Model file for the job. Use its own axes, mm. A direction names the side the tool comes from. Give positions to 0.01 mm unless a question says otherwise; leave off trailing zeros. Loops run counter-clockwise (first coordinate to the right, second up) from the corner with the lowest first, then second, coordinate; pieces in that order, holes last. Notation, with made-up numbers: M 86,33 L 104,33 A10 cw 104,37 Z; hole C -15.75,12 d10. An arc over 180 degrees is marked long. Use CSV: the item, a comma, the result in double quotes. Start each with the question number.
(1) Flat gauge pins, fed straight in: P1, Ø3, axis at y = 4, z = -2, coming from the -X side; P2, Ø3, axis at y = 4, z = -4, coming from the +X side; P3, Ø1.5, axis at x = 14.5, z = -34, coming from the -Y side; P4, Ø3, axis at x = 3, y = 3, coming from the -Z side. Where does each tip first touch, or does it go through?
(2) Two-plate mould, pull along X, no slides. Class faces 5 (the face through (73, 3, -6.35)), 6 (the face through (88.9, 3, -25)), 7 (the face through (47, 6.35, -64)), 8 (the face through (0, 3, -38)): pulls with the +X half, pulls with the -X half, needs draft (parallel to the pull), parting line crosses it, or undercut.
(3) Slice it at A-A on x = 49. List the corners of the cut face in (y, z).
(4) Wall check: line 1 along Z through (x, y) = (53, 0.5); line 2 along X through (y, z) = (3.25, -105.5). Give the ranges that are in metal, low to high. Write a range as from..to.
(5) Slice it at B-B on z = -105.5. List the corners of the cut face in (x, y).
(6) Tool access for faces 1 (the face through (6.35, 3, -124)), 2 (the face through (6.35, 3, -76)), 3 (the face through (88.9, 3, -102)), 4 (the face through (15.875, 3, -124)): list every direction of +Z, -Z, +X, -X, +Y, -Y with a clear straight run to the whole face (end or side of a thin tool).
```python
from build123d import *

# Parameters (mm, degrees)
SKETCH1_W           = 95.25
SKETCH1_H           = 127
BOSS_EXTRUDE1_DEPTH = 6.35
SKETCH2_W           = 6.35
SKETCH2_H           = 12.7
SKETCH2_H_2         = 6.35
CUT_EXTRUDE1_DEPTH  = 7.35
LPATTERN1_COUNT     = 5
LPATTERN1_PITCH     = 25.4
SKETCH4_W           = 12.7
SKETCH4_H           = 6.35
CUT_EXTRUDE3_DEPTH  = 7.35
LPATTERN2_COUNT     = 2
LPATTERN2_PITCH     = 25.4
LPATTERN2_COL_COUNT = 2
LPATTERN2_COL_PITCH = 25.4


with BuildPart() as part:
    # Sketch1 → Boss-Extrude1 (new body)
    with BuildSketch(Plane(origin=(0, 0, 0), x_dir=(1, 0, 0), z_dir=(0, 1, 0))):
        with Locations((47.625, 63.5)):
            Rectangle(SKETCH1_W, SKETCH1_H)
    extrude(amount=BOSS_EXTRUDE1_DEPTH)

    # Sketch2 → Cut-Extrude1 (cut, through all)
    with BuildSketch(Plane(origin=(0, 6.35, 0), x_dir=(1, 0, 0), z_dir=(0, 1, 0))):
        with Locations((3.175, 127)):
            Rectangle(SKETCH2_W, SKETCH2_H)
        with Locations((92.075, 127)):
            Rectangle(SKETCH2_W, SKETCH2_H)
        with Locations((3.175, 3.175)):
            Rectangle(SKETCH2_W, SKETCH2_H_2)
        with Locations((92.075, 3.175)):
            Rectangle(SKETCH2_W, SKETCH2_H_2)
    cut_extrude1 = extrude(amount=-CUT_EXTRUDE1_DEPTH, mode=Mode.SUBTRACT)

    # LPattern1: Cut-Extrude1 ×5
    with Locations(*[(0, 0, i * LPATTERN1_PITCH) for i in range(1, LPATTERN1_COUNT)]):
        add(cut_extrude1, mode=Mode.SUBTRACT)

    # Sketch4 → Cut-Extrude3 (cut, through all)
    with BuildSketch(Plane(origin=(0, 6.35, 0), x_dir=(1, 0, 0), z_dir=(0, 1, 0))):
        with Locations((47.625, 123.825)):
            Rectangle(SKETCH4_W, SKETCH4_H)
        with Locations((47.625, 3.175)):
            Rectangle(SKETCH4_W, SKETCH4_H)
    cut_extrude3 = extrude(amount=-CUT_EXTRUDE3_DEPTH, mode=Mode.SUBTRACT)

    # LPattern2: Cut-Extrude3 ×2
    with Locations(*[(-i * LPATTERN2_PITCH, 0, 0) for i in range(1, LPATTERN2_COUNT)]):
        add(cut_extrude3, mode=Mode.SUBTRACT)

    # LPattern2 col: Cut-Extrude3 ×2
    with Locations(*[(i * LPATTERN2_COL_PITCH, 0, 0) for i in range(1, LPATTERN2_COL_COUNT)]):
        add(cut_extrude3, mode=Mode.SUBTRACT)


solid = part.part
```
Reply:
1,P1,"stops at x = 6.35"
1,P2,"stops at x = 88.9"
1,P3,"stops at y = 0"
1,P4,"stops at z = -120.65"
2,face 5,"undercut"
2,face 6,"pulls with the +X half"
2,face 7,"needs draft"
2,face 8,"pulls with the -X half"
3,outline,"M 0,-120.65 L 6.35,-120.65 L 6.35,-6.35 L 0,-6.35 Z"
4,line 1,"z = -120.65..-6.35"
4,line 2,"x = 6.35..88.9"
5,outline,"M 6.35,0 L 88.9,0 L 88.9,6.35 L 6.35,6.35 Z"
6,face 1,"-Z, -X, +Y, -Y"
6,face 2,"-X, +Y, -Y"
6,face 3,"+X, +Y, -Y"
6,face 4,"-Z, +Y, -Y"
